Geometry check sheet. Reference: the model listing, model coordinates, mm. A direction names the side the tool comes from. Give positions to 0.01 mm unless a question says otherwise; leave off trailing zeros. Loops run counter-clockwise (first coordinate to the right, second up) from the corner with the lowest first, then second, coordinate; pieces in that order, holes last. Notation, with made-up numbers: (44, 68) - (103, 68) arc R18 cw to (103, 102) - close; hole circle Ø3 at (-8.5, 88). An arc over 180 degrees is marked (long way). Use a Markdown table: item, result. Add a question column.
1. Cross-section at B-B on z = 0. Enter the section's corners in (x, y).
2. Material ranges on L1, parallel to Y at x = 0.75, z = 6.75; L2, parallel to Z at x = 3.5, y = -16; L3, parallel to Y at x = 3.75, z = 4.75, recorded low to high.
3. Depth check by flat-ended pin: P1, Ø10, axis at x = -3.5, y = -18.5, coming from the +Z side; P2, Ø10, axis at y = -8.5, z = -1.5, coming from the +X side; P3, Ø5, axis at y = -16.5, z = 9.5, coming from the -X side; P4, Ø2, axis at x = -2, y = -20.5, coming from the -Z side. Enter the tip coordinate at first touch or a pass-through.
4. Cross-section at A-A on x = 0. Enter the section's corners in (y, z).
5. Cross-section at C-C on y = -21. Enter the section's corners in (x, z), and give its area (3 significant figures).
6. Cross-section at D-D on x = -8. Enter the section's corners in (y, z).
7. Set-up check for faces 1 (the cylindrical face through (-1.38, -24.42, -6.2)), 2 (the flat face through (7.152, 3.131, 8.383)): record each of +Z, -Z, +X, -X, +Y, -Y from which the full face is reachable in a straight line by a thin tool's end or side.
from build123d import *

# Parameters (mm, degrees)
F0_R     = 6.35
F1_DEPTH = 50.8
F3_DEPTH = 6.35
F4_SIZE  = 1.27


with BuildPart() as f1:
    # F0 (on Front) → F1 (new body)
    with BuildSketch(Plane.XZ):
        Circle(F0_R)
    extrude(amount=F1_DEPTH)

    # F2 (on Front) → F3 (join)
    with BuildSketch(Plane.XZ):
        Polygon((-10.933553, -3.694675), (-4.831777, -10.16), (4.058223, -10.16), (10.16, -3.694675), (10.16, 5.195325), (4.058223, 11.660649), (-4.831777, 11.660649), (-10.933553, 5.195325), align=None)
    extrude(amount=-F3_DEPTH)

    # F4
    f4_edges = [f1.edges().sort_by_distance(p)[0] for p in [
        (-6.35, -50.8, 0),
    ]]
    chamfer(f4_edges, length=F4_SIZE)


solid = f1.part
Values found:
| question | item | result |
|---|---|---|
| 1 | outline | (-10.93, 0) - (-6.35, 0) - (-6.35, -49.53) - (-5.08, -50.8) - (5.08, -50.8) - (6.35, -49.53) - (6.35, 0) - (10.16, 0) - (10.16, 6.35) - (-10.93, 6.35) - close |
| 2 | L1 | y = 0 to 6.35 |
| 2 | L2 | z = -5.3 to 5.3 |
| 2 | L3 | y = -49.83 to 6.35 |
| 3 | P1 | stops at z = 6.35 |
| 3 | P2 | stops at x = 6.35 |
| 3 | P3 | passes through |
| 3 | P4 | stops at z = -6.27 |
| 4 | outline | (-50.8, -5.08) - (-49.53, -6.35) - (0, -6.35) - (0, -10.16) - (6.35, -10.16) - (6.35, 11.66) - (0, 11.66) - (0, 6.35) - (-49.53, 6.35) - (-50.8, 5.08) - close |
| 5 | outline | circle Ø12.7 at (0, 0) |
| 5 | area | 127 mm2 |
| 6 | outline | (0, -6.8) - (6.35, -6.8) - (6.35, 8.3) - (0, 8.3) - close |
| 7 | face 1 | -Y |
| 7 | face 2 | +Z, +X, +Y, -Y |
